Input: part model. Units: mm. Frame: model coordinates. A direction names the side the tool comes from. Coordinates: 2 decimals unless noted, no trailing zeros. Loops run counter-clockwise (first coordinate to the right, second up) from the corner with the lowest first, then second, coordinate; pieces in that order, holes last. Notation, with made-up numbers: M 40,-25.5 L 45,-25.5 A38 ccw 45,12.5 Z; hole C 1,53 d11. An arc over 180 degrees is marked long. Use a Markdown table: item, result. Add a question column.
1. Section C-C on y = 3.6. Output: boundary loops of the cut face in (x, z).
2. Draft query along Z for faces 4 (the flat face through (-3.1, 4.5, 3.1)), 5 (the cylindrical face through (0.9, 2.46, 2.86)), 6 (the cylindrical face through (0.33, 2.465, -7.493)), 7 (the flat face through (1, 0, -3)). Return one class per face: +Z half, -Z half, draft (parallel to the pull), parting line (faces both ways), or undercut.
3. Section A-A on x = 0. Output: boundary loops of the cut face in (y, z).
4. Line query: L1, parallel to X at y = 4.7, z = 0; L2, parallel to X at y = 0.35, z = 0; L3, parallel to X at y = 2.25, z = 0. Output: solid intervals per line, ascending. Write a range as [from, to].
5. Section D-D on z = 6. Output: boundary loops of the cut face in (x, y), then the cut area to 3 significant figures.
6. Pin query (flat end, axial travel): pin 1 (3 mm diameter, centred on x = -2.5, y = 2.5, fed in from -Z); pin 2 (2 mm diameter, centred on x = 4, y = 3.5, fed in from +Z); pin 3 (1 mm diameter, centred on x = -2, y = 1.5, fed in from -Z). Return the tip coordinate at first contact, or that it passes through.
7. Section B-B on z = 0. Output: boundary loops of the cut face in (x, y), then the cut area to 3 significant figures.
8. Set-up query: faces 1 (the flat face through (-3, 0.5, -3)), 2 (the flat face through (-7, 0, 2)), 3 (the cylindrical face through (1.242, 4.754, 3.944)). Return all of +Z, -Z, +X, -X, +Y, -Y with unobstructed straight access to the full face (end or side cutting, diameter ignored); none if empty.
```python
from build123d import *

# Parameters (mm, degrees)
CROQUIS1_R              = 7.5
CROQUIS1_R_2            = 3
SALIENTE_EXTRUIR1_DEPTH = 5
CROQUIS2_R              = 7.124900464
CROQUIS2_R_2            = 4.13518393
CORTAR_EXTRUIR1_DEPTH   = 0.5
CROQUIS3_R              = 6.927022016
CROQUIS3_R_2            = 3.541649153
CORTAR_EXTRUIR2_DEPTH   = 0.5


with BuildPart() as part:
    # Croquis1 → Saliente-Extruir1 (new body)
    with BuildSketch(Plane(origin=(0, 0, 0), x_dir=(1, 0, 0), z_dir=(0, 1, 0))):
        with Locations(Location((0, 0, 0), (0, 0, 270))):
            Circle(CROQUIS1_R)
        with Locations(Location((0, 0, 0), (0, 0, 270))):
            Circle(CROQUIS1_R_2, mode=Mode.SUBTRACT)
    extrude(amount=SALIENTE_EXTRUIR1_DEPTH)

    # Croquis2 → Cortar-Extruir1 (cut)
    with BuildSketch(Plane(origin=(0, 5, 0), x_dir=(1, 0, 0), z_dir=(0, 1, 0))):
        with Locations(Location((0, 0, 0), (0, 0, 270))):
            Circle(CROQUIS2_R)
        with Locations(Location((0, 0, 0), (0, 0, 270))):
            Circle(CROQUIS2_R_2, mode=Mode.SUBTRACT)
    extrude(amount=-CORTAR_EXTRUIR1_DEPTH, mode=Mode.SUBTRACT)

    # Croquis3 → Cortar-Extruir2 (cut)
    with BuildSketch(Plane.XZ):
        with Locations(Location((0, 0, 0), (0, 0, 270))):
            Circle(CROQUIS3_R)
        with Locations(Location((0, 0, 0), (0, 0, 270))):
            Circle(CROQUIS3_R_2, mode=Mode.SUBTRACT)
    extrude(amount=-CORTAR_EXTRUIR2_DEPTH, mode=Mode.SUBTRACT)


solid = part.part
```
Answers below:
| question | item | result |
|---|---|---|
| 1 | outline | C 0,0 d15; hole C 0,0 d6 |
| 2 | face 4 | undercut |
| 2 | face 5 | undercut |
| 2 | face 6 | parting line |
| 2 | face 7 | draft |
| 3 | outline | M 0,-7.5 L 5,-7.5 L 5,-7.12 L 4.5,-7.12 L 4.5,-4.14 L 5,-4.14 L 5,-3 L 0,-3 L 0,-3.54 L 0.5,-3.54 L 0.5,-6.93 L 0,-6.93 Z; M 0,3 L 5,3 L 5,4.14 L 4.5,4.14 L 4.5,7.12 L 5,7.12 L 5,7.5 L 0,7.5 L 0,6.93 L 0.5,6.93 L 0.5,3.54 L 0,3.54 Z |
| 4 | L1 | x = [-7.5, -7.12], [-4.14, -3], [3, 4.14], [7.12, 7.5] |
| 4 | L2 | x = [-7.5, -6.93], [-3.54, -3], [3, 3.54], [6.93, 7.5] |
| 4 | L3 | x = [-7.5, -3], [3, 7.5] |
| 5 | outline | M -4.5,0 L -3.46,0 L -3.46,0.5 L 3.46,0.5 L 3.46,0 L 4.5,0 L 4.5,5 L 3.84,5 L 3.84,4.5 L -3.84,4.5 L -3.84,5 L -4.5,5 Z |
| 5 | area | 37.7 mm² |
| 6 | pin 1 | stops at z = -7.43 |
| 6 | pin 2 | stops at z = 6.87 |
| 6 | pin 3 | stops at z = -7.35 |
| 7 | outline | M -7.5,0 L -6.93,0 L -6.93,0.5 L -3.54,0.5 L -3.54,0 L -3,0 L -3,5 L -4.14,5 L -4.14,4.5 L -7.12,4.5 L -7.12,5 L -7.5,5 Z; M 3,0 L 3.54,0 L 3.54,0.5 L 6.93,0.5 L 6.93,0 L 7.5,0 L 7.5,5 L 7.12,5 L 7.12,4.5 L 4.14,4.5 L 4.14,5 L 3,5 Z |
| 7 | area | 38.6 mm² |
| 8 | face 1 | -Y |
| 8 | face 2 | +Z, -Z, +X, -X, -Y |
| 8 | face 3 | +Y |
